For this review, use the dimensioned drawing (mm, ordinates from the lowest corner) and the shaded views. Round coordinates to 2 decimals unless told otherwise and drop trailing zeros. Loops run counter-clockwise (first coordinate to the right, second up) from the corner with the lowest first, then second, coordinate; pieces in that order, holes last.
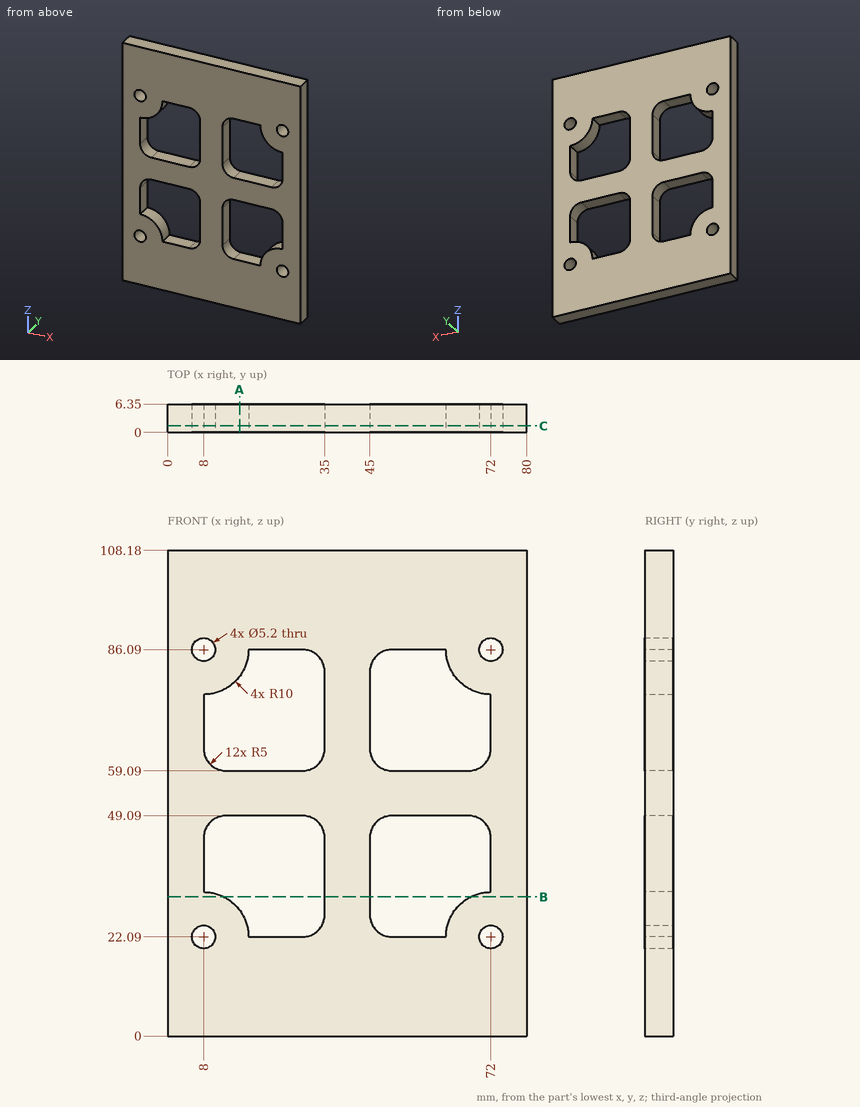
(1) Add section C-C (y = 1.5). Give the number of separate pieces and of enclosed holes in the cut face, plus the area to 3 significant figures.
(2) For L1, parallel to X at y = 0.75, z = 36; L2, parallel to Z at x = 25, y = 3.5; L3, parallel to Z at x = 64, y = 3.75, list the stretches that pass through material, from the lowest coordinate up.
(3) Add section B-B (z = 31). Give the boundary of the cut face in (x, y).
(4) Add section A-A (x = 16). Give the boundary of the cut face in (y, z), plus the area to 3 significant figures.
Outcome:
1. separate pieces: 1
1. enclosed holes: 8
1. area: 6,030 mm2
2. L1: x = 0 to 8, 35 to 45, 72 to 80
2. L2: z = 0 to 22.09, 49.09 to 59.09, 86.09 to 108.18
2. L3: z = 0 to 28.09, 49.09 to 59.09, 80.09 to 108.18
3. outline: (0, 0) - (12.54, 0) - (12.54, 6.35) - (0, 6.35) - close; (35, 0) - (45, 0) - (45, 6.35) - (35, 6.35) - close; (67.46, 0) - (80, 0) - (80, 6.35) - (67.46, 6.35) - close
4. outline: (0, 0) - (6.35, 0) - (6.35, 28.09) - (0, 28.09) - close; (0, 49.09) - (6.35, 49.09) - (6.35, 59.09) - (0, 59.09) - close; (0, 80.09) - (6.35, 80.09) - (6.35, 108.18) - (0, 108.18) - close
4. area: 420 mm2
